from build123d import *

# Parameters (mm, degrees)
SKETCH1_W           = 108
SKETCH1_H           = 108
BOSS_EXTRUDE1_DEPTH = 10
FILLET1_R           = 5
FILLET3_R           = 2


with BuildPart() as part:
    # Sketch1 → Boss-Extrude1 (new body)
    with BuildSketch(Plane(origin=(0, 0, 0), x_dir=(1, 0, 0), z_dir=(0, 1, 0))):
        Rectangle(SKETCH1_W, SKETCH1_H)
        Polygon((-42, 47), (-42, 37), (-47, 37), (-47, 5), (-35, 5), (-5, 35), (-5, 47), align=None, mode=Mode.SUBTRACT)
        Polygon((-32.928932188, 0), (0, 32.928932188), (32.928932188, 0), (0, -32.928932188), align=None, mode=Mode.SUBTRACT)
        Polygon((5, 47), (5, 35), (35, 5), (47, 5), (47, 42), (37, 42), (37, 47), align=None, mode=Mode.SUBTRACT)
        Polygon((47, -5), (35, -5), (5, -35), (5, -47), (42, -47), (42, -37), (47, -37), align=None, mode=Mode.SUBTRACT)
        Polygon((-5, -47), (-5, -35), (-35, -5), (-47, -5), (-47, -42), (-37, -42), (-37, -47), align=None, mode=Mode.SUBTRACT)
    extrude(amount=BOSS_EXTRUDE1_DEPTH)

    # Fillet1
    fillet1_edges = [part.edges().sort_by_distance(p)[0] for p in [
        (-5, 5, -35),
        (-5, 5, -47),
        (-42, 5, -47),
        (-47, 5, -5),
        (-35, 5, -5),
        (-32.928932188, 5, 0),
        (0, 5, 32.928932188),
        (32.928932188, 5, 0),
        (0, 5, -32.928932188),
        (5, 5, -35),
        (35, 5, -5),
        (47, 5, -5),
        (47, 5, -42),
        (5, 5, -47),
        (35, 5, 5),
        (5, 5, 35),
        (5, 5, 47),
        (42, 5, 47),
        (47, 5, 5),
        (-5, 5, 35),
        (-35, 5, 5),
        (-47, 5, 5),
        (-47, 5, 42),
        (-5, 5, 47),
    ]]
    fillet(fillet1_edges, radius=FILLET1_R)

    # Fillet3
    fillet3_edges = [part.edges().sort_by_distance(p)[0] for p in [
        (-42, 5, -37),
        (-47, 5, -37),
        (37, 5, -42),
        (37, 5, -47),
        (42, 5, 37),
        (47, 5, 37),
        (-37, 5, 42),
        (-37, 5, 47),
    ]]
    fillet(fillet3_edges, radius=FILLET3_R)


solid = part.part
The model under review builds one solid part; all positions refer to its coordinate system, in mm. Round coordinates to 2 decimals unless told otherwise and drop trailing zeros. Loops run counter-clockwise (first coordinate to the right, second up) from the corner with the lowest first, then second, coordinate; pieces in that order, holes last. Notation, with made-up numbers: M -38,-24 L -10,-24 A28 cw -10,12 Z; hole C 51.25,-13 d7. An arc over 180 degrees is marked long. Answer as CSV lines item,"result". Start each with the question number.
Item 1: Wall thickness on line 1 (Z direction, x = 22, y = 2.75); line 2 (X direction, y = 2.5, z = -9); line 3 (Z direction, x = 20, y = 1.5): over which ranges is each line inside the solid? List them lowest first. Write a range as [from, to].
Item 2: Mouldability with a two-part tool opening along Z and no side actions: class faces 1 (the face through (-5, 5, -40)), 2 (the face through (23, 0, -13)) as released by +Z, released by -Z, zero draft, split by the parting line, or undercut.
Item 3: Consider section C-C (y = 8.5). State how many separate pieces and enclosed holes the cut face has, then the cut area to 3 significant figures.
Item 4: Consider section B-B (z = 20.5). Write out the cut boundary in (x, y).
Item 5: Consider section A-A (x = 17.5). Write out the cut boundary in (y, z).
Answer:
1,line 1,"z = [-54, -47], [-18, -10.93], [10.93, 18], [47, 54]"
1,line 2,"x = [-54, -46.9], [-31, -23.93], [23.93, 31], [46.9, 54]"
1,line 3,"z = [-54, -47], [-20, -12.93], [12.93, 20], [47, 54]"
2,face 1,"undercut"
2,face 2,"zero draft"
3,separate pieces,"1"
3,enclosed holes,"5"
3,area,"4,530 mm^2"
4,outline,"M -54,0 L -47,0 L -47,10 L -54,10 Z; M -19.5,0 L -12.43,0 L -12.43,10 L -19.5,10 Z; M 12.43,0 L 19.5,0 L 19.5,10 L 12.43,10 Z; M 47,0 L 54,0 L 54,10 L 47,10 Z"
5,outline,"M 0,-54 L 10,-54 L 10,-47 L 0,-47 Z; M 0,-22.5 L 10,-22.5 L 10,-15.43 L 0,-15.43 Z; M 0,15.43 L 10,15.43 L 10,22.5 L 0,22.5 Z; M 0,47 L 10,47 L 10,54 L 0,54 Z"
